```python
from build123d import *

# Parameters (mm, degrees)
SKETCH1_R           = 2.413
BOSS_EXTRUDE1_DEPTH = 44.45
SKETCH2_R           = 2.413
CUT_EXTRUDE1_DEPTH  = 50.8
SKETCH3_W           = 44.45
SKETCH3_H           = 25.654
CUT_EXTRUDE2_DEPTH  = 77.989658396
SKETCH4_R           = 14.2875
CUT_EXTRUDE3_DEPTH  = 6.35


with BuildPart() as part:
    # Sketch1 → Boss-Extrude1 (new body)
    with BuildSketch(Plane(origin=(0, 0, 0), x_dir=(1, 0, 0), z_dir=(0, 1, 0))):
        Polygon((0, 38.1), (6.35, 44.45), (38.1, 44.45), (44.45, 38.1), (44.45, 6.35), (38.1, 0), (6.35, 0), (0, 6.35), align=None)
        with Locations(Location((9.525, 22.225, 0), (0, 0, 270))):
            Circle(SKETCH1_R, mode=Mode.SUBTRACT)
        with Locations(Location((22.225, 22.225, 0), (0, 0, 270))):
            Circle(SKETCH1_R, mode=Mode.SUBTRACT)
        with Locations(Location((34.925, 22.225, 0), (0, 0, 270))):
            Circle(SKETCH1_R, mode=Mode.SUBTRACT)
    extrude(amount=BOSS_EXTRUDE1_DEPTH)

    # Sketch2 → Cut-Extrude1 (cut)
    with BuildSketch(Plane(origin=(44.45, 0, 0), x_dir=(0, 0, -1), z_dir=(1, 0, 0))):
        with Locations((9.525, 31.75)):
            Circle(SKETCH2_R)
        with Locations((34.925, 31.75)):
            Circle(SKETCH2_R)
        with Locations((34.925, 12.7)):
            Circle(SKETCH2_R)
        with Locations((9.525, 12.7)):
            Circle(SKETCH2_R)
    extrude(amount=-CUT_EXTRUDE1_DEPTH, mode=Mode.SUBTRACT)

    # Sketch3 → Cut-Extrude2 (cut, through all)
    with BuildSketch(Plane(origin=(44.45, 0, 0), x_dir=(0, 0, -1), z_dir=(1, 0, 0))):
        with Locations((22.225, 31.623)):
            Rectangle(SKETCH3_W, SKETCH3_H)
    extrude(amount=-CUT_EXTRUDE2_DEPTH, mode=Mode.SUBTRACT)

    # Sketch4 → Cut-Extrude3 (cut)
    with BuildSketch(Plane.XY):
        with Locations((22.225, 25.4)):
            Circle(SKETCH4_R)
    cut_extrude3 = extrude(amount=-CUT_EXTRUDE3_DEPTH, mode=Mode.SUBTRACT)

    # Mirror1: Cut-Extrude3 across plane
    add(cut_extrude3.mirror(Plane.XY.offset(-22.225)), mode=Mode.SUBTRACT)


solid = part.part
```
Read the model definition and answer for the solid it produces. Units are mm, in the model's axes. A direction names the side the tool comes from. Give positions to 0.01 mm unless a question says otherwise; leave off trailing zeros. Order: outer loops, then holes, each group sorted by start corner. A loop starts at its lowest first (then second) coordinate and runs counter-clockwise, first axis right, second up.
(1) Find section B-B (x = 11). Give the vertices of the cut face in (y, z) (3 decimals), plus the area to 3 significant figures.
(2) Straight lines are drawn through the part: L1, parallel to X at y = 17.25, z = -22; L2, parallel to X at y = 13, z = -23; L3, parallel to Z at x = 8, y = 13.5. For each, find the intervals that lie inside material, in ascending order.
(3) Find section A-A (y = 12.7). Give the vertices of the cut face in (x, z) (3 decimals), plus the area to 3 significant figures.
(4) Find section C-C (z = -8). Give the vertices of the cut face in (x, y).
(5) Given pin 1 (3 mm diameter, centred on x = 17.5, z = -8.5, fed in from -Y); pin 2 (1.5 mm diameter, centred on x = 39.5, y = 12, fed in from +Z); pin 3 (2 mm diameter, centred on x = 40, y = 17, fed in from +Z); pin 4 (4 mm diameter, centred on x = 18, y = 14, fed in from +Z), each flat-ended and moving along its own axis, determine where each tip first touches the part or whether it passes through.
(6) For faces 4 (the cylindrical face through (22.007, 11.114, -3.131)), 5 (the cylindrical face through (35.031, 9.266, -24.636)), 6 (the flat face through (22, 16, -38.1)), determine the directions among +Z, -Z, +X, -X, +Y, -Y from which every point of the face is accessible in a straight line to the end or side of a thin tool.
(7) Find section D-D (x = 40.5). Give the vertices of the cut face in (y, z) (3 decimals), plus the area to 3 significant figures.
(8) For a pull along X with two mould halves and no side action, classify faces 1 (the cylindrical face through (9.631, 9.266, -24.636)), 2 (the flat face through (0, 9, -22)), 3 (the flat face through (41.3, 9.3, -3.2)) as released by +X, released by -X, zero draft, split by the parting line, or undercut.
Result sheet:
1. outline: (0, -44.45) - (16.561, -44.45) - (16.561, -38.1) - (18.796, -38.1) - (18.796, -24.135) - (0, -24.135) - close; (0, -20.315) - (18.796, -20.315) - (18.796, -6.35) - (16.561, -6.35) - (16.561, 0) - (0, 0) - close; hole circle Ø4.826 at (12.7, -34.925); hole circle Ø4.826 at (12.7, -9.525)
1. area: 699 mm2
2. L1: x = 0 to 7.12, 11.93 to 19.82, 24.63 to 32.52, 37.33 to 44.45
2. L2: x = 0 to 7.24, 11.81 to 19.94, 24.51 to 32.64, 37.21 to 44.45
2. L3: z = -44.45 to -37.2, -32.65 to -24.1, -20.35 to -11.8, -7.25 to 0
3. outline: (0, -38.1) - (6.35, -44.45) - (15.68, -44.45) - (15.68, -38.1) - (28.77, -38.1) - (28.77, -44.45) - (38.1, -44.45) - (44.45, -38.1) - (44.45, -37.338) - (0, -37.338) - close; (0, -32.512) - (44.45, -32.512) - (44.45, -11.938) - (0, -11.938) - close; (0, -7.112) - (44.45, -7.112) - (44.45, -6.35) - (38.1, 0) - (28.77, 0) - (28.77, -6.35) - (15.68, -6.35) - (15.68, 0) - (6.35, 0) - (0, -6.35) - close; hole circle Ø4.826 at (9.525, -22.225); hole circle Ø4.826 at (22.225, -22.225); hole circle Ø4.826 at (34.925, -22.225)
3. area: 1,240 mm2
4. outline: (0, 0) - (44.45, 0) - (44.45, 10.83) - (0, 10.83) - close; (0, 14.57) - (44.45, 14.57) - (44.45, 18.8) - (0, 18.8) - close
5. pin 1: stops at y = 0
5. pin 2: stops at z = -0.65
5. pin 3: stops at z = -0.9
5. pin 4: stops at z = -6.35
6. face 4: +Z, +Y
6. face 5: +Y, -Y
6. face 6: -Z, +Y
7. outline: (0, -42.05) - (18.796, -42.05) - (18.796, -2.4) - (0, -2.4) - close; hole circle Ø4.826 at (12.7, -34.925); hole circle Ø4.826 at (12.7, -9.525)
7. area: 709 mm2
8. face 1: undercut
8. face 2: released by -X
8. face 3: released by +X
